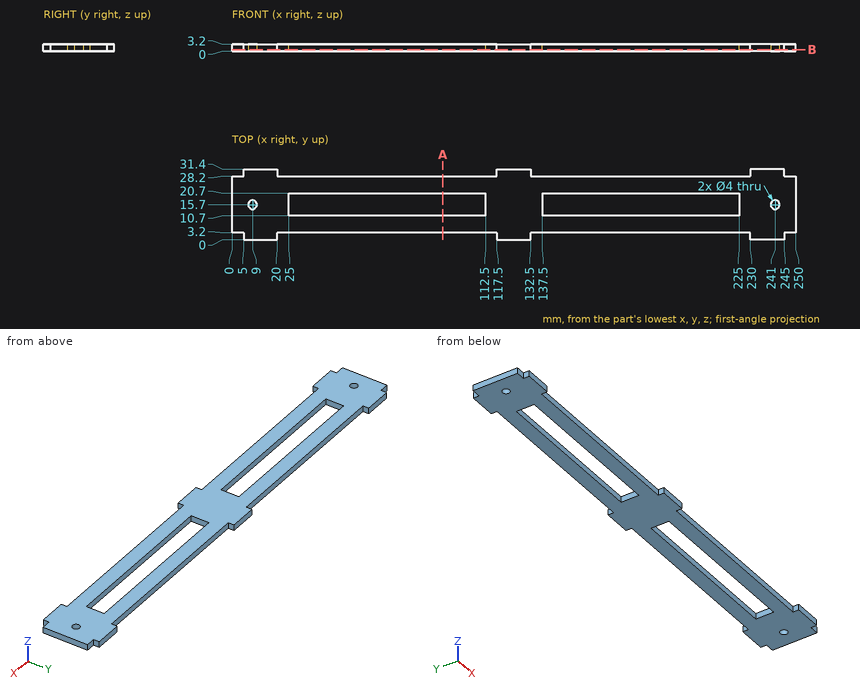
Geometry check sheet. Reference: drawing and pictorial views, mm from the part's lowest x, y, z. Round coordinates to 2 decimals unless told otherwise and drop trailing zeros. Loops run counter-clockwise (first coordinate to the right, second up) from the corner with the lowest first, then second, coordinate; pieces in that order, holes last.
1. Scan lines: probe 1 along X at (y, z) = (12.5, 2.65); probe 2 along X at (y, z) = (16, 2.6); probe 3 along Y at (x, z) = (174, 1.85). Record each from-to range of solid material in increasing order.
2. Sectioned sample at A-A on x = 93.5. Record the boundary of the cut face in (y, z).
3. Sectioned sample at B-B on z = 0.75. Give the number of separate pieces and of enclosed holes in the cut face, and give its area (3 significant figures).
4. Gauge pin test, flat ends, axial feed: pin 1 Ø1.6 at (y, z) = (30, 2.5) entering from +X; pin 2 Ø5 at (x, y) = (71, 21.5) entering from -Z; pin 3 Ø1.6 at (x, z) = (247.5, 2) entering from -Y; pin 4 Ø1.6 at (x, z) = (66, 1) entering from +Y. Record the tip position at first contact, or that the pin passes through.
Recorded:
1. probe 1: x = 0 to 25, 112.5 to 137.5, 225 to 250
1. probe 2: x = 0 to 7.02, 10.98 to 25, 112.5 to 137.5, 225 to 239.02, 242.98 to 250
1. probe 3: y = 3.2 to 10.7, 20.7 to 28.2
2. outline: (3.2, 0) - (10.7, 0) - (10.7, 3.2) - (3.2, 3.2) - close; (20.7, 0) - (28.2, 0) - (28.2, 3.2) - (20.7, 3.2) - close
3. separate pieces: 1
3. enclosed holes: 4
3. area: 4,760 mm2
4. pin 1: stops at x = 245
4. pin 2: stops at z = 0
4. pin 3: stops at y = 3.2
4. pin 4: stops at y = 28.2
